Verification items for the finished model (mm, model axes). A direction names the side the tool comes from. Round coordinates to 2 decimals unless told otherwise and drop trailing zeros. Loops run counter-clockwise (first coordinate to the right, second up) from the corner with the lowest first, then second, coordinate; pieces in that order, holes last. Notation, with made-up numbers: M 85,-11.75 L 128,-11.75 A27 cw 128,27.25 Z; hole C 64.25,72 d10. An arc over 180 degrees is marked long. One line per item, written item: value.
from build123d import *

# Parameters (mm, degrees)
SKETCH1_W           = 200
SKETCH1_H           = 250
BOSS_EXTRUDE1_DEPTH = 5
SKETCH2_W           = 200
SKETCH2_H           = 250
SKETCH2_W_2         = 190
SKETCH2_H_2         = 240
BOSS_EXTRUDE2_DEPTH = 70
BOSS_EXTRUDE3_START = -15
SKETCH3_W           = 190
SKETCH3_H           = 240
BOSS_EXTRUDE3_DEPTH = 5
SKETCH4_R           = 25
CUT_EXTRUDE1_DEPTH  = 5


with BuildPart() as part:
    # Sketch1 → Boss-Extrude1 (new body)
    with BuildSketch(Plane.XY):
        with Locations((100, -125)):
            Rectangle(SKETCH1_W, SKETCH1_H)
    extrude(amount=BOSS_EXTRUDE1_DEPTH)

    # Sketch2 → Boss-Extrude2 (add)
    with BuildSketch(Plane.XY.offset(5)):
        with Locations((100, -125)):
            Rectangle(SKETCH2_W, SKETCH2_H)
        with Locations((100, -125)):
            Rectangle(SKETCH2_W_2, SKETCH2_H_2, mode=Mode.SUBTRACT)
    extrude(amount=BOSS_EXTRUDE2_DEPTH)

    # Sketch3 → Boss-Extrude3 (add)
    with BuildSketch(Plane.XY.offset(75).offset(BOSS_EXTRUDE3_START)):
        with Locations((100, -125)):
            Rectangle(SKETCH3_W, SKETCH3_H)
    extrude(amount=BOSS_EXTRUDE3_DEPTH)

    # Sketch4 → Cut-Extrude1 (cut)
    with BuildSketch(Plane.XY.offset(65)):
        with Locations((35, -35)):
            Circle(SKETCH4_R)
        with Locations((95, -35)):
            Circle(SKETCH4_R)
        with Locations((155, -35)):
            Circle(SKETCH4_R)
        with Locations((95, -95)):
            Circle(SKETCH4_R)
        with Locations((155, -95)):
            Circle(SKETCH4_R)
        with Locations((95, -155)):
            Circle(SKETCH4_R)
        with Locations((155, -155)):
            Circle(SKETCH4_R)
        with Locations((95, -215)):
            Circle(SKETCH4_R)
        with Locations((155, -215)):
            Circle(SKETCH4_R)
        with Locations((35, -95)):
            Circle(SKETCH4_R)
        with Locations((35, -155)):
            Circle(SKETCH4_R)
        with Locations((35, -215)):
            Circle(SKETCH4_R)
    extrude(amount=-CUT_EXTRUDE1_DEPTH, mode=Mode.SUBTRACT)


solid = part.part
(1) Sectioned sample at D-D on x = 125. Enter the section's corners in (y, z).
Completed:
outline: M -250,0 L 0,0 L 0,75 L -5,75 L -5,65 L -245,65 L -245,75 L -250,75 Z; hole M -245,5 L -5,5 L -5,60 L -245,60 Z
(2) Sectioned sample at B-B on y = -215. Enter the section's corners in (x, z), and give its area (3 significant figures).
Completed:
outline: M 0,0 L 200,0 L 200,75 L 195,75 L 195,65 L 180,65 L 180,60 L 195,60 L 195,5 L 5,5 L 5,60 L 10,60 L 10,65 L 5,65 L 5,75 L 0,75 Z; M 60,60 L 70,60 L 70,65 L 60,65 Z; M 120,60 L 130,60 L 130,65 L 120,65 Z
area: 1,900 mm^2
(3) Sectioned sample at C-C on z = 41. Enter the section's corners in (x, y), and give its area (3 significant figures).
Completed:
outline: M 0,-250 L 200,-250 L 200,0 L 0,0 Z; hole M 5,-245 L 195,-245 L 195,-5 L 5,-5 Z
area: 4,400 mm^2
(4) Mould release check, pull along X, two halves, no side actions. Record for faces 1 (the face through (91.745, -190.213, 62.535)), 2 (the face through (200, -127, 37)), 3 (the face through (99, 0, 37)): +X half, -X half, draft (parallel to the pull), parting line (faces both ways), or undercut.
Completed:
face 1: undercut
face 2: +X half
face 3: draft
(5) Thickness scan on L1, parallel to Y at x = 95, z = 61; L2, parallel to X at y = -176, z = 35.5; L3, parallel to Z at x = 150, y = -126. Record the ranges inside material, lowest first. Write a range as from..to.
Completed:
L1: y = -250..-240, -190..-180, -130..-120, -70..-60, -10..0
L2: x = 0..5, 195..200
L3: z = 0..5, 60..65
(6) Tool access check on faces 4 (the face through (195, -127, 32)), 5 (the face through (75, -110, 63)), 6 (the face through (0, -127, 37)). Record the directions out of +Z, -Z, +X, -X, +Y, -Y that give a thin tool (end or side, any length) a straight path to the whole face; none if there is none.
Completed:
face 4: none
face 5: +Z
face 6: +Z, -Z, -X, +Y, -Y
(7) Depth check by flat-ended pin: pin 1 Ø5 at (x, y) = (134.5, -213.5) entering from +Z. Enter the tip coordinate at first touch or a pass-through.
Completed:
pin 1: stops at z = 5
(8) Sectioned sample at A-A on x = 20. Enter the section's corners in (y, z), and give its area (3 significant figures).
Completed:
outline: M -250,0 L 0,0 L 0,75 L -5,75 L -5,65 L -15,65 L -15,60 L -5,60 L -5,5 L -245,5 L -245,60 L -235,60 L -235,65 L -245,65 L -245,75 L -250,75 Z; M -195,60 L -175,60 L -175,65 L -195,65 Z; M -135,60 L -115,60 L -115,65 L -135,65 Z; M -75,60 L -55,60 L -55,65 L -75,65 Z
area: 2,350 mm^2
